```python
from build123d import *

# Parameters (mm, degrees)
SKETCH1_W           = 25.4
SKETCH1_H           = 25.4
BOSS_EXTRUDE1_DEPTH = 12.7
SKETCH2_W           = 25.4
SKETCH2_H           = 6.35
BOSS_EXTRUDE2_DEPTH = 12.7
SKETCH6_W           = 2.925
SKETCH6_H           = 10.16
BOSS_EXTRUDE3_DEPTH = 18.288
SKETCH8_W           = 1.27
SKETCH8_H           = 8.255
SKETCH8_H_2         = 10.16
BOSS_EXTRUDE4_DEPTH = 11.938
SKETCH9_W           = 25.4
SKETCH9_H           = 2.286
BOSS_EXTRUDE5_DEPTH = 11.938
SKETCH10_R          = 1.9939
CUT_EXTRUDE1_DEPTH  = 34.777225226
CUT_EXTRUDE2_DEPTH  = 43.17693142


with BuildPart() as part:
    # Sketch1 → Boss-Extrude1 (new body)
    with BuildSketch(Plane(origin=(0, 0, 0), x_dir=(1, 0, 0), z_dir=(0, 1, 0))):
        Rectangle(SKETCH1_W, SKETCH1_H)
    extrude(amount=BOSS_EXTRUDE1_DEPTH)

    # Sketch2 → Boss-Extrude2 (add)
    with BuildSketch(Plane.ZY.offset(12.7)):
        with Locations((0, 3.175)):
            Rectangle(SKETCH2_W, SKETCH2_H)
    boss_extrude2 = extrude(amount=BOSS_EXTRUDE2_DEPTH)

    # Mirror1: Boss-Extrude2 across plane
    add(boss_extrude2.mirror(Plane(origin=(0, 0, 0), x_dir=(0, 0, 1), z_dir=(1, 0, 0))))

    # Sketch6 → Boss-Extrude3 (add)
    with BuildSketch(Plane(origin=(0, 6.35, 0), x_dir=(1, 0, 0), z_dir=(0, 1, 0))):
        with Locations((-14.1625, 5.17)):
            Rectangle(SKETCH6_W, SKETCH6_H)
        with Locations((14.1625, 5.17)):
            Rectangle(SKETCH6_W, SKETCH6_H)
    extrude(amount=BOSS_EXTRUDE3_DEPTH)

    # Sketch8 → Boss-Extrude4 (add)
    with BuildSketch(Plane(origin=(0, 12.7, 0), x_dir=(1, 0, 0), z_dir=(0, 1, 0))):
        with Locations((-12.065, 4.2175)):
            Rectangle(SKETCH8_W, SKETCH8_H)
        with Locations((12.065, 5.17)):
            Rectangle(SKETCH8_W, SKETCH8_H_2)
    extrude(amount=BOSS_EXTRUDE4_DEPTH)

    # Sketch9 → Boss-Extrude5 (add)
    with BuildSketch(Plane(origin=(0, 12.7, 0), x_dir=(1, 0, 0), z_dir=(0, 1, 0))):
        with Locations((0, -11.557)):
            Rectangle(SKETCH9_W, SKETCH9_H)
    extrude(amount=BOSS_EXTRUDE5_DEPTH)

    # Sketch10 → Cut-Extrude1 (cut, through all)
    with BuildSketch(Plane(origin=(0, 6.35, 0), x_dir=(1, 0, 0), z_dir=(0, 1, 0))):
        with Locations(Location((21.59, -2.54, 0), (0, 0, 270))):
            Circle(SKETCH10_R)
        with Locations(Location((-21.59, -2.54, 0), (0, 0, 270))):
            Circle(SKETCH10_R)
    extrude(amount=-CUT_EXTRUDE1_DEPTH, mode=Mode.SUBTRACT)

    # Sketch11 → Cut-Extrude2 (cut, through all)
    with BuildSketch(Plane(origin=(0, 0, -10.25), x_dir=(-1, 0, 0), z_dir=(0, 0, -1))):
        with BuildLine():
            ThreePointArc((15.125, 18.8), (15.090925826, 19.058819045), (14.991025404, 19.3))
            ThreePointArc((14.991025404, 19.3), (13.125, 18.8), (14.991025404, 18.3))
            ThreePointArc((14.991025404, 18.3), (15.090925826, 18.541180955), (15.125, 18.8))
        make_face()
        with BuildLine():
            ThreePointArc((-14.991025404, 19.3), (-15.125, 18.8), (-14.991025404, 18.3))
            ThreePointArc((-14.991025404, 18.3), (-13.866180955, 17.834074174), (-13.125, 18.8))
            ThreePointArc((-13.125, 18.8), (-13.866180955, 19.765925826), (-14.991025404, 19.3))
        make_face()
    extrude(amount=-CUT_EXTRUDE2_DEPTH, mode=Mode.SUBTRACT)


solid = part.part
```
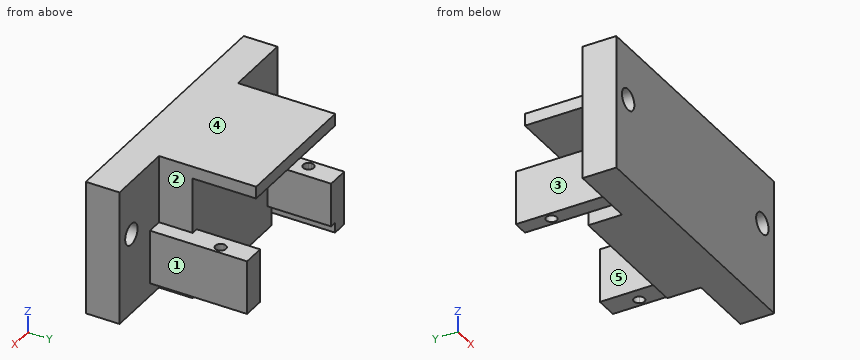
For this review, take the finished solid that the model builds, in its own axes (mm). Face numbers are marked on the shaded views. A direction names the side the tool comes from. Round coordinates to 2 decimals unless told otherwise and drop trailing zeros. Write each loop counter-clockwise with the first axis right and the second up, starting at its lowest first coordinate (ties: lowest second). Pieces come first, ordered by that corner, then holes. Notation, with made-up numbers: M 68.5,46 L 113.5,46 A20 ccw 113.5,77 Z; hole C 43,88.5 d4. An arc over 180 degrees is marked long. One line per item, written item: value. Start each with the question number.
(1) We need section D-D (z = 8). Give the boundary of the cut face in (x, y).
(2) We need section C-C (z = -6.75). Give the boundary of the cut face in (x, y) (3 decimals).
(3) Wall thickness on line 1 (Y direction, x = -15, z = 2.75); line 2 (Y direction, x = 6.5, z = -9.75); line 3 (Z direction, x = -15.5, y = 19.25): over which ranges is each line inside the solid? List them lowest first.
(4) We need section A-A (x = 21.59). Give the boundary of the cut face in (y, z), and give its area (3 significant figures).
(5) Insertion check: pin 1 (4 mm diameter, centred on x = -14, y = 15.5, fed in from -Z); pin 2 (5 mm diameter, centred on x = -10.5, z = 7.5, fed in from +Y); pin 3 (8 mm diameter, centred on y = 11.5, z = 2, fed in from +X) (3 decimals). Each pin has a flat end and moves straight along its axis. Give the tip position at first contact, or say it passes through.
(6) We need section B-B (y = 16.5). Give the boundary of the cut face in (x, z) (3 decimals).
(7) Machinability: for the marked faces 1, 2, 3, 4 and 5, which of the approach directions +Z, -Z, +X, -X, +Y, -Y give a long, thin tool a straight path to every point of the face, cutting with its end or side? Answer none if there is none.
Result:
1. outline: M -25.4,0 L 25.4,0 L 25.4,6.35 L 12.7,6.35 L 12.7,12.7 L -12.7,12.7 L -12.7,6.35 L -25.4,6.35 Z
2. outline: M -25.4,0 L 25.4,0 L 25.4,6.35 L 15.625,6.35 L 15.625,24.638 L 11.43,24.638 L 11.43,12.7 L -11.43,12.7 L -11.43,24.638 L -15.625,24.638 L -15.625,6.35 L -25.4,6.35 Z; hole C -14.125,18.8 d2; hole C 14.125,18.8 d2
3. line 1: 0 to 6.35
3. line 2: 0 to 12.7
3. line 3: -10.25 to -0.09
4. outline: M 0,-12.7 L 6.35,-12.7 L 6.35,0.55 L 0,0.55 Z; M 0,4.53 L 6.35,4.53 L 6.35,12.7 L 0,12.7 Z
4. area: 136 mm²
5. pin 1: z = -10.25
5. pin 2: y = 12.7
5. pin 3: x = 15.625
6. outline: M -15.625,-10.25 L -12.7,-10.25 L -12.7,-8.345 L -11.43,-8.345 L -11.43,-0.09 L -15.625,-0.09 Z; M -12.7,10.414 L 12.7,10.414 L 12.7,12.7 L -12.7,12.7 Z; M 11.43,-10.25 L 15.625,-10.25 L 15.625,-0.09 L 11.43,-0.09 Z
7. face 1: +Z, -Z, +X, +Y
7. face 2: +Z, +X, +Y
7. face 3: +Z, -Z, -X, +Y
7. face 4: +Z, +X, -X, +Y, -Y
7. face 5: -Z, +Y
